Input: part model. Units: mm. Frame: model coordinates. Round coordinates to 2 decimals unless told otherwise and drop trailing zeros. Order: outer loops, then holes, each group sorted by start corner. A loop starts at its lowest first (then second) coordinate and runs counter-clockwise, first axis right, second up.
Item 1: Cut plane B-B on x = -56. Output: boundary loops of the cut face in (y, z) (3 decimals).
Item 2: First-contact query: pin 1 (1 mm diameter, centred on x = -24, z = 1, fed in from -Y). Flat tip, straight axial feed; report the tip coordinate or a pass-through.
Item 3: Cut plane A-A on z = 0.7. Output: boundary loops of the cut face in (x, y).
Item 4: Line query: L1, parallel to Y at x = -46.5, z = 0.3; L2, parallel to X at y = -15.5, z = 0.45; L3, parallel to X at y = -16.25, z = 2.9. Output: solid intervals per line, ascending.
Autodesk Inventor part; units mm, degrees
ref_plane "YZ Plane" through (0, 0, 0) normal (1, 0, 0) x (0, 1, 0)
ref_plane "XZ Plane" through (0, 0, 0) normal (0, 1, 0) x (-1, 0, 0)
ref_plane "XY Plane" through (0, 0, 0) normal (0, 0, 1) x (1, 0, 0)
sketch "Sketch1" plane through (0, 0, 0) normal (0, 0, 1) x (1, 0, 0)
  line L0 (-86.188, -1.6122) -> (142.412, -1.6122)
  line L1 (142.412, -1.6122) -> (142.412, -14.3122)
  line L2 (142.412, -14.3122) -> (57.4807, -14.3122)
  line L3 (-86.188, -14.3122) -> (-86.188, -1.6122)
  line L4 (53.512, -18.2809) -> (53.512, -18.2809)
  line L5 (53.512, -18.2809) -> (40.812, -18.2809)
  line L6 (40.812, -18.2809) -> (40.812, -18.2809)
  line L7 (36.8432, -14.3122) -> (-86.188, -14.3122)
  arc A0 (40.812, -18.2809) -> (36.8432, -14.3122) centre (36.8432, -18.2809) ccw
  arc A1 (57.4807, -14.3122) -> (53.512, -18.2809) centre (57.4807, -18.2809) ccw
  point P0 (0, 0)
  point P1 (53.512, -14.3122)
  dimension "d0" = 228.6
  dimension "d1" = 12.7
  dimension "d2" = 12.7
  dimension "d3" = 3.9688
  dimension "d4" = 88.9
  dimension "d5" = 3.9688
extrude "Extrusion1" add sketch "Sketch1" along normal blind 3.175
properties part number "Granny Gearbox Routing Template Horizontal Tabs"
From the geometry:
1. outline: (-14.312, 0) - (-1.612, 0) - (-1.612, 3.175) - (-14.312, 3.175) - close
2. pin 1: stops at y = -14.31
3. outline: (-86.19, -14.31) - (36.84, -14.31) arc R3.97 cw to (40.81, -18.28) - (53.51, -18.28) arc R3.97 cw to (57.48, -14.31) - (142.41, -14.31) - (142.41, -1.61) - (-86.19, -1.61) - close
4. L1: y = -14.31 to -1.61
4. L2: x = 39.67 to 54.65
4. L3: x = 40.25 to 54.07
